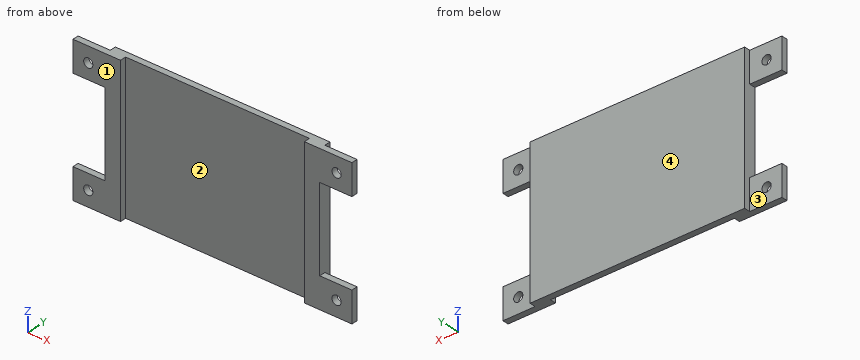
```python
from build123d import *

# Parameters (mm, degrees)
SKETCH1_R           = 3
BOSS_EXTRUDE1_DEPTH = 8
SKETCH2_W           = 21
SKETCH2_H           = 20
CUT_EXTRUDE1_DEPTH  = 4
SKETCH3_W           = 120
SKETCH3_H           = 95
CUT_EXTRUDE2_DEPTH  = 4


with BuildPart() as part:
    # Sketch1 → Boss-Extrude1 (new body)
    with BuildSketch(Plane(origin=(0, 0, 0), x_dir=(1, 0, 0), z_dir=(0, 1, 0))):
        Polygon((0, 0), (21, 0), (161, 0), (182, 0), (182, -20), (161, -20), (161, -75), (182, -75), (182, -95), (0, -95), (0, -75), (21, -75), (21, -20), (0, -20), align=None)
        with Locations(Location((10, -10, 0), (0, 0, 270))):
            Circle(SKETCH1_R, mode=Mode.SUBTRACT)
        with Locations(Location((10, -85, 0), (0, 0, 270))):
            Circle(SKETCH1_R, mode=Mode.SUBTRACT)
        with Locations(Location((172, -10, 0), (0, 0, 90))):
            Circle(SKETCH1_R, mode=Mode.SUBTRACT)
        with Locations(Location((172, -85, 0), (0, 0, 90))):
            Circle(SKETCH1_R, mode=Mode.SUBTRACT)
    extrude(amount=BOSS_EXTRUDE1_DEPTH)

    # Sketch2 → Cut-Extrude1 (cut)
    with BuildSketch(Plane(origin=(0, 8, 0), x_dir=(1, 0, 0), z_dir=(0, 1, 0))):
        with Locations((10.5, -85)):
            Rectangle(SKETCH2_W, SKETCH2_H)
        with Locations((10.5, -10)):
            Rectangle(SKETCH2_W, SKETCH2_H)
        with Locations((171.5, -85)):
            Rectangle(SKETCH2_W, SKETCH2_H)
        with Locations((171.5, -10)):
            Rectangle(SKETCH2_W, SKETCH2_H)
    extrude(amount=-CUT_EXTRUDE1_DEPTH, mode=Mode.SUBTRACT)

    # Sketch3 → Cut-Extrude2 (cut)
    with BuildSketch(Plane.XZ):
        with Locations((91, 47.5)):
            Rectangle(SKETCH3_W, SKETCH3_H)
    extrude(amount=-CUT_EXTRUDE2_DEPTH, mode=Mode.SUBTRACT)


solid = part.part
```
Source: CAD feature listing. Evaluate the final solid. Frame: model axes, mm. Face numbers are marked on the shaded views. A direction names the side the tool comes from. Give positions to 0.01 mm unless a question says otherwise; leave off trailing zeros. Loops run counter-clockwise (first coordinate to the right, second up) from the corner with the lowest first, then second, coordinate; pieces in that order, holes last. Notation, with made-up numbers: (53, -29) - (93, -29) arc R17 ccw to (93, -24) - close; hole circle Ø2 at (10, -13.5). An arc over 180 degrees is marked (long way). Use CSV: the item, a comma, the result in double quotes. Start each with the question number.
1. Section D-D (x = 104). Output: boundary loops of the cut face in (y, z).
2. Section C-C (z = 69.5). Output: boundary loops of the cut face in (x, y).
3. Section B-B (z = 10). Output: boundary loops of the cut face in (x, y), then the cut area to 3 significant figures.
4. Ray query, L1, parallel to X at y = 2.35, z = 10; L2, parallel to Z at x = 10, y = 2.4; L3, parallel to X at y = 2.25, z = 70. Return the intervals inside material, ascending.
5. Pin query (flat end, axial travel): pin 1 (10 mm diameter, centred on x = 11.5, z = 82, fed in from +Y); pin 2 (4 mm diameter, centred on y = 3.5, z = 44.5, fed in from +X); pin 3 (2.5 mm diameter, centred on y = 2.5, z = 66.5, fed in from -X). Return the tip coordinate at first contact, or that it passes through.
6. Reachability of the marked faces 3 and 4 from +Z, -Z, +X, -X, +Y, -Y: full face, straight path, thin tool, end or side. Return the list, or none.
7. Draft query along X for the marked faces 1 and 2. Return one class per face: +X half, -X half, draft (parallel to the pull), parting line (faces both ways), or undercut.
8. Section A-A (x = 172). Output: boundary loops of the cut face in (y, z), then the cut area to 3 significant figures.
Response:
1,outline,"(4, 0) - (8, 0) - (8, 95) - (4, 95) - close"
2,outline,"(21, 0) - (31, 0) - (31, 4) - (151, 4) - (151, 0) - (161, 0) - (161, 8) - (21, 8) - close"
3,outline,"(0, 0) - (7, 0) - (7, 4) - (0, 4) - close; (13, 0) - (31, 0) - (31, 4) - (151, 4) - (151, 0) - (169, 0) - (169, 4) - (161, 4) - (161, 8) - (21, 8) - (21, 4) - (13, 4) - close; (175, 0) - (182, 0) - (182, 4) - (175, 4) - close"
3,area,"760 mm²"
4,L1,"0 to 7, 13 to 31, 151 to 169, 175 to 182"
4,L2,"0 to 7, 13 to 20, 75 to 82, 88 to 95"
4,L3,"21 to 31, 151 to 161"
5,pin 1,"y = 4"
5,pin 2,"x = 161"
5,pin 3,"x = 21"
6,face 3,"+Z, -Z, -X, +Y"
6,face 4,"+Z, -Z, +X, -X, +Y"
7,face 1,"draft"
7,face 2,"undercut"
8,outline,"(0, 0) - (4, 0) - (4, 7) - (0, 7) - close; (0, 13) - (4, 13) - (4, 20) - (0, 20) - close; (0, 75) - (4, 75) - (4, 82) - (0, 82) - close; (0, 88) - (4, 88) - (4, 95) - (0, 95) - close"
8,area,"112 mm²"
